Geometry: final body of the model. Coordinates: model frame, mm. A direction names the side the tool comes from. Give positions to 0.01 mm unless a question says otherwise; leave off trailing zeros. Write each loop counter-clockwise with the first axis right and the second up, starting at its lowest first coordinate (ties: lowest second). Pieces come first, ordered by that corner, then holes. Notation, with made-up numbers: (7, 46) -> (14, 46) arc R25 cw to (14, 76) -> close; hole circle Ø6 at (56.5, -8). An arc over 180 degrees is marked (long way). Answer as a JSON object with one key per item and string values. Group by question number.
(1) Draft query along Y for faces 1 (the face through (0, 13, 450)), 2 (the face through (15, 5, 222)), 3 (the face through (0, 33, 222)), 4 (the face through (0, 0, 222)). Return one class per face: +Y half, -Y half, draft (parallel to the pull), parting line (faces both ways), or undercut.
(2) Section query B-B on y = 25. Output: boundary loops of the cut face in (x, z), plus the area to 3 significant figures.
(3) Material intervals for probe 1 along X at (y, z) = (3.9, 225) (3 decimals); probe 2 along Z at (x, y) = (13.5, 4.5); probe 3 along Z at (x, y) = (-13, 4), sorted ascending.
(4) Set-up query: faces 5 (the face through (0, 13, 0)), 6 (the face through (-15, 5, 222)). Return all of +Z, -Z, +X, -X, +Y, -Y with unobstructed straight access to the full face (end or side cutting, diameter ignored); none if empty.
(5) Section query A-A on z = 116.5. Output: boundary loops of the cut face in (x, y).
(6) Contact query for flat-ended pins moving along their axis: pin 1 Ø3 at (x, z) = (-15, 276.5) entering from +Y; pin 2 Ø0.5 at (x, z) = (9, 204) entering from +Y; pin 3 Ø4 at (x, z) = (-5, 98.5) entering from +Y. Output: stop coordinate, or through.
from build123d import *

# Parameters (mm, degrees)
BOSS_EXTRUDE1_DEPTH = 450
SKETCH2_R           = 2.75
CUT_EXTRUDE1_DEPTH  = 450


with BuildPart() as part:
    # Sketch1 → Boss-Extrude1 (new body)
    with BuildSketch(Plane.XY):
        with BuildLine():
            Line((20, 0), (-20, 0))
            Line((-20, 0), (-20, 5))
            Line((-20, 5), (-9.25, 5))
            Line((-9.25, 5), (-9.25, 11.7))
            Line((-9.25, 11.7), (-8.605626905, 11.7))
            Line((-8.605626905, 11.7), (-3.487119155, 17.8))
            ThreePointArc((-3.487119155, 17.8), (0, 33), (3.487119155, 17.8))
            Line((3.487119155, 17.8), (8.605626905, 11.7))
            Line((8.605626905, 11.7), (9.25, 11.7))
            Line((9.25, 11.7), (9.25, 5))
            Line((9.25, 5), (20, 5))
            Line((20, 5), (20, 0))
        make_face()
    extrude(amount=BOSS_EXTRUDE1_DEPTH)

    # Sketch2 → Cut-Extrude1 (cut)
    with BuildSketch(Plane(origin=(0, 0, 0), x_dir=(1, 0, 0), z_dir=(0, 1, 0))):
        with Locations((-14.625, -75)):
            Circle(SKETCH2_R)
        with Locations(Location((14.625, -75, 0), (0, 0, 90))):
            Circle(SKETCH2_R)
        with Locations((-14.625, -225)):
            Circle(SKETCH2_R)
        with Locations(Location((14.625, -225, 0), (0, 0, 90))):
            Circle(SKETCH2_R)
        with Locations((-14.625, -375)):
            Circle(SKETCH2_R)
        with Locations(Location((14.625, -375, 0), (0, 0, 90))):
            Circle(SKETCH2_R)
    extrude(amount=CUT_EXTRUDE1_DEPTH, mode=Mode.SUBTRACT)


solid = part.part
Answer list:
{
 "1": {"face 1": "draft", "face 2": "+Y half", "face 3": "undercut", "face 4": "-Y half"},
 "2": {"outline": "(-8, 0) -> (8, 0) -> (8, 450) -> (-8, 450) -> close", "area": "7,200 mm2"},
 "3": {"probe 1": "-20 to -17.375, -11.875 to 11.875, 17.375 to 20", "probe 2": "0 to 72.49, 77.51 to 222.49, 227.51 to 372.49, 377.51 to 450", "probe 3": "0 to 72.78, 77.22 to 222.78, 227.22 to 372.78, 377.22 to 450"},
 "4": {"face 5": "-Z, +X, -X, +Y, -Y", "face 6": "+Z, -Z, -X, +Y"},
 "5": {"outline": "(-20, 0) -> (20, 0) -> (20, 5) -> (9.25, 5) -> (9.25, 11.7) -> (8.61, 11.7) -> (3.49, 17.8) arc R8 ccw (long way) to (-3.49, 17.8) -> (-8.61, 11.7) -> (-9.25, 11.7) -> (-9.25, 5) -> (-20, 5) -> close"},
 "6": {"pin 1": "y = 5", "pin 2": "y = 11.7", "pin 3": "y = 32.42"}
}
